Source: CAD feature listing. Evaluate the final solid. Frame: model axes, mm. A direction names the side the tool comes from. Give positions to 0.01 mm unless a question says otherwise; leave off trailing zeros. Write each loop counter-clockwise with the first axis right and the second up, starting at its lowest first coordinate (ties: lowest second). Pieces come first, ordered by that corner, then holes. Notation, with made-up numbers: M 15,3.5 L 37,3.5 A12 cw 37,17.5 Z; hole C 41.25,31 d7. An arc over 180 degrees is marked long. Use CSV: the item, a comma, the result in double quotes. Start each with the question number.
from build123d import *

# Parameters (mm, degrees)
SM_BASE_FLANGE_1_DEPTH   = 3
OTHER_START              = -9
OTHER_1_DEPTH            = 18
HOLE_WIZARD_2_AT_2_COUNT = 2
HOLE_WIZARD_2_AT_2_PITCH = 24


# Read off the part's stored shape, not the designer's step: 褶边1
# Sheet-metal steps are written as plain solids
with BuildPart() as part:
    # Sketch 1 → 基体-法兰1 (new body)
    with BuildSketch(Plane(origin=(0, 0, 0), x_dir=(1, 0, 0), z_dir=(0, 1, 0))):
        with BuildLine():
            Line((-9.5, -13.5), (9.5, -13.5))
            Line((9.5, -13.5), (9.5, -8.5))
            Line((9.5, -8.5), (25, -8.5))
            Line((25, -8.5), (25, 6.5))
            ThreePointArc((25, 6.5), (23.535533906, 10.035533906), (20, 11.5))
            Line((20, 11.5), (-20, 11.5))
            ThreePointArc((-20, 11.5), (-23.535533906, 10.035533906), (-25, 6.5))
            Line((-25, 6.5), (-25, -8.5))
            Line((-25, -8.5), (-9.5, -8.5))
            Line((-9.5, -8.5), (-9.5, -13.5))
        make_face()
    extrude(amount=-SM_BASE_FLANGE_1_DEPTH)

    # Other 1 outline → Other 1 (add)
    with BuildSketch(Plane.YZ.offset(OTHER_START)):
        with BuildLine():
            Line((2, 11.5), (2, 8.5))
            ThreePointArc((2, 8.5), (5.535533906, 17.035533906), (-3, 13.5))
            Line((-3, 13.5), (0, 13.5))
            ThreePointArc((0, 13.5), (3.414213562, 14.914213562), (2, 11.5))
        make_face()
    extrude(amount=OTHER_1_DEPTH)

    # 草图13 → 打孔尺寸(%根据十字)槽半沉头木螺钉的类型2 (revolve, cut)
    with BuildSketch(Plane(origin=(-12, 0, 0), x_dir=(0, 0, 1), z_dir=(1, 0, 0))):
        Polygon((0, 0), (0, 3), (2.25, 3), (2.25, 2.05), (4.3, 0), align=None)
    hole_wizard_2 = revolve(axis=Axis((-12, 6.35, 0), (0, -1, 0)), mode=Mode.SUBTRACT)

    # 打孔尺寸(%根据十字)槽半沉头木螺钉的类型2 at 2: 打孔尺寸(%根据十字)槽半沉头木螺钉的类型2 ×2
    with Locations(*[(i * HOLE_WIZARD_2_AT_2_PITCH, 0, 0) for i in range(1, HOLE_WIZARD_2_AT_2_COUNT)]):
        add(hole_wizard_2, mode=Mode.SUBTRACT)


solid = part.part
Item 1: Material intervals for probe 1 along X at (y, z) = (-2.7, 0); probe 2 along Z at (x, y) = (12, -2.6); probe 3 along Y at (x, z) = (-7, -5), sorted ascending.
Item 2: Pull-direction query (X, two-part tool) for faces 1 (the conical face through (14.32, -1.92, -0.52)), 2 (the flat face through (25, -1, 1)), 3 (the flat face through (0, -1, -11.5)); classes: released by +X, released by -X, zero draft, split by the parting line, or undercut.
Item 3: Section D-D (x = 18). Return the cut outline in (y, z), plus the area to 3 significant figures.
Item 4: Section C-C (z = -6). Return the cut outline in (x, y).
Item 5: Section A-A (x = -12). Return the cut outline in (y, z).
Item 6: Contact query for flat-ended pins moving along their axis: pin 1 Ø1.5 at (y, z) = (0, 13) entering from +X; pin 2 Ø5 at (x, z) = (12, 0) entering from +Y; pin 3 Ø1.5 at (x, y) = (18.5, -1.5) entering from +Z; pin 4 Ø4 at (x, z) = (-12, 0) entering from +Y. Output: stop coordinate, or through.
Item 7: Set-up query: faces 4 (the flat face through (9.5, -1, 11)), 5 (the flat face through (9, 4, 15)), 6 (the flat face through (0, 2, 10)), 7 (the flat face through (-9.5, -1, 11)), 8 (the flat face through (-9, 4, 15)). Return all of +Z, -Z, +X, -X, +Y, -Y with unobstructed straight access to the full face (end or side cutting, diameter ignored); none if empty.
Item 8: Section B-B (z = 0). Return the cut outline in (x, y).
Output values:
1,probe 1,"x = -25 to -14.25, -9.75 to 9.75, 14.25 to 25"
1,probe 2,"z = -11.5 to -2.25, 2.25 to 8.5"
1,probe 3,"y = -3 to 0"
2,face 1,"undercut"
2,face 2,"released by +X"
2,face 3,"zero draft"
3,outline,"M -3,-11.5 L 0,-11.5 L 0,8.5 L -3,8.5 Z"
3,area,"60.0 mm2"
4,outline,"M -25,-3 L 25,-3 L 25,0 L -25,0 Z"
5,outline,"M -3,-11.5 L 0,-11.5 L 0,-4.3 L -2.05,-2.25 L -3,-2.25 Z; M -3,2.25 L -2.05,2.25 L 0,4.3 L 0,8.5 L -3,8.5 Z"
6,pin 1,"stops at x = 9.5"
6,pin 2,"stops at y = -1.8"
6,pin 3,"stops at z = 8.5"
6,pin 4,"passes through"
7,face 4,"+Z, +X, +Y, -Y"
7,face 5,"+Z, +X, +Y"
7,face 6,"-Z, +X, -X"
7,face 7,"+Z, -X, +Y, -Y"
7,face 8,"+Z, -X, +Y"
8,outline,"M -25,-3 L -14.25,-3 L -14.25,-2.05 L -16.3,0 L -25,0 Z; M -9.75,-3 L 9.75,-3 L 9.75,-2.05 L 7.7,0 L -7.7,0 L -9.75,-2.05 Z; M 14.25,-3 L 25,-3 L 25,0 L 16.3,0 L 14.25,-2.05 Z"
